from build123d import *

# Parameters (mm, degrees)
SKETCH1_R           = 6
BOSS_EXTRUDE1_DEPTH = 6


with BuildPart() as part:
    # Sketch1 → Boss-Extrude1 (new body)
    with BuildSketch(Plane.XY):
        Polygon((-211.428617248, -75.762954902), (-211.428617248, -105.762954902), (-202.683627049, -105.762954902), (-202.683627049, -111.762954902), (-202.683627049, -117.762954902), (-182.683627049, -117.762954902), (-182.683627049, -111.762954902), (-182.683627049, -105.762954902), (-174.549373808, -105.762954902), (-174.549373808, -75.762954902), (-182.683627049, -75.762954902), (-182.683627049, -69.762954902), (-182.683627049, -63.762954902), (-202.683627049, -63.762954902), (-202.683627049, -69.762954902), (-202.683627049, -75.762954902), align=None)
        with Locations((-192.988995528, -90.762954902)):
            Circle(SKETCH1_R, mode=Mode.SUBTRACT)
    extrude(amount=BOSS_EXTRUDE1_DEPTH)


solid = part.part
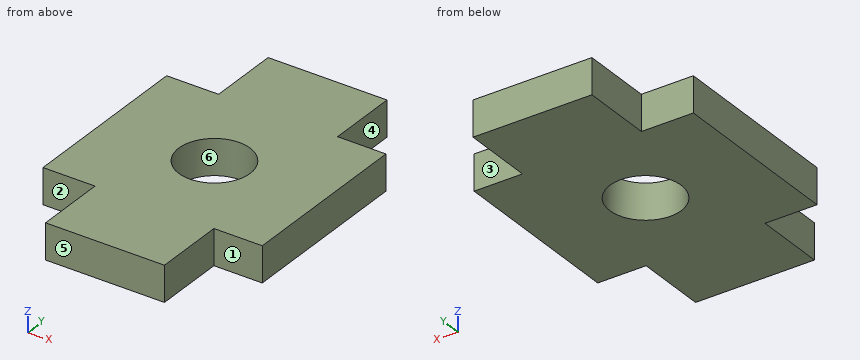
Read the model definition and answer for the solid it produces. Units are mm, in the model's axes. Face numbers are marked on the shaded views. A direction names the side the tool comes from. Round coordinates to 2 decimals unless told otherwise and drop trailing zeros. Order: outer loops, then holes, each group sorted by start corner. A loop starts at its lowest first (then second) coordinate and runs counter-clockwise, first axis right, second up.
1) The mould has two halves that part along X. Classify the marked faces 4, 5 and 6: released by +X, released by -X, zero draft, split by the parting line, or undercut.
2) For the marked faces 1, 2 and 3, determine the directions among +Z, -Z, +X, -X, +Y, -Y from which every point of the face is accessible in a straight line to the end or side of a thin tool.
3) The part is cut by section D-D on y = -72. Write down the section's boundary in (x, z), plus the area to 3 significant figures.
4) The part is cut by section B-B on z = 3.55. Write down the section's boundary in (x, y).
5) Straight lines are drawn through the part: L1, parallel to X at y = -71, z = 1.1; L2, parallel to X at y = -92, z = 5.2; L3, parallel to X at y = -90, z = 3. For each, find the intervals that lie inside material, in ascending order.
6) The part is cut by section A-A on y = -89.5. Write down the section's boundary in (x, z).
7) Flat-ended cylindrical pins translate along their axes: pin 1 (3 mm diameter, centred on y = -71, z = 4, fed in from +X); pin 2 (1 mm diameter, centred on x = -205.5, z = 2.5, fed in from -Y); pin 3 (3 mm diameter, centred on y = -111, z = 3.5, fed in from -X). Find the tip coordinate at first contact, or state that the pin passes through.
8) The part is cut by section C-C on x = -195.5. Write down the section's boundary in (y, z).
Resolved:
1. face 4: released by +X
1. face 5: zero draft
1. face 6: undercut
2. face 1: +Z, -Z, +X, -Y
2. face 2: +Z, -Z, -X, -Y
2. face 3: +Z, -Z, +X, +Y
3. outline: (-202.68, 0) - (-182.68, 0) - (-182.68, 6) - (-202.68, 6) - close
3. area: 120 mm2
4. outline: (-211.43, -105.76) - (-202.68, -105.76) - (-202.68, -117.76) - (-182.68, -117.76) - (-182.68, -105.76) - (-174.55, -105.76) - (-174.55, -75.76) - (-182.68, -75.76) - (-182.68, -63.76) - (-202.68, -63.76) - (-202.68, -75.76) - (-211.43, -75.76) - close; hole circle Ø12 at (-192.99, -90.76)
5. L1: x = -202.68 to -182.68
5. L2: x = -211.43 to -198.86, -187.12 to -174.55
5. L3: x = -211.43 to -198.94, -187.04 to -174.55
6. outline: (-211.43, 0) - (-198.85, 0) - (-198.85, 6) - (-211.43, 6) - close; (-187.12, 0) - (-174.55, 0) - (-174.55, 6) - (-187.12, 6) - close
7. pin 1: stops at x = -182.68
7. pin 2: stops at y = -105.76
7. pin 3: stops at x = -202.68
8. outline: (-117.76, 0) - (-96.21, 0) - (-96.21, 6) - (-117.76, 6) - close; (-85.31, 0) - (-63.76, 0) - (-63.76, 6) - (-85.31, 6) - close
